```python
from build123d import *

# Parameters (mm, degrees)
SKETCH1_W           = 116
SKETCH1_H           = 79
SKETCH1_W_2         = 112
SKETCH1_H_2         = 75
BOSS_EXTRUDE1_DEPTH = 24
SKETCH2_W           = 116
SKETCH2_H           = 79
BOSS_EXTRUDE2_DEPTH = 2
SKETCH3_W           = 73
SKETCH3_H           = 48
CUT_EXTRUDE1_DEPTH  = 2
SKETCH4_R           = 1.75
CUT_EXTRUDE2_DEPTH  = 2
SKETCH6_R           = 7
CUT_EXTRUDE3_DEPTH  = 10
CUT_EXTRUDE4_DEPTH  = 2
SKETCH8_R           = 5
CUT_EXTRUDE5_DEPTH  = 2


with BuildPart() as part:
    # Sketch1 → Boss-Extrude1 (new body)
    with BuildSketch(Plane(origin=(0, 0, 0), x_dir=(1, 0, 0), z_dir=(0, 1, 0))):
        Rectangle(SKETCH1_W, SKETCH1_H)
        Rectangle(SKETCH1_W_2, SKETCH1_H_2, mode=Mode.SUBTRACT)
    extrude(amount=BOSS_EXTRUDE1_DEPTH)

    # Sketch2 → Boss-Extrude2 (add)
    with BuildSketch(Plane(origin=(0, 24, 0), x_dir=(1, 0, 0), z_dir=(0, 1, 0))):
        Rectangle(SKETCH2_W, SKETCH2_H)
    extrude(amount=BOSS_EXTRUDE2_DEPTH)

    # Sketch3 → Cut-Extrude1 (cut)
    with BuildSketch(Plane(origin=(0, 26, 0), x_dir=(1, 0, 0), z_dir=(0, 1, 0))):
        Rectangle(SKETCH3_W, SKETCH3_H)
    extrude(amount=-CUT_EXTRUDE1_DEPTH, mode=Mode.SUBTRACT)

    # Sketch4 → Cut-Extrude2 (cut)
    with BuildSketch(Plane(origin=(0, 26, 0), x_dir=(1, 0, 0), z_dir=(0, 1, 0))):
        with Locations((50, -27.5)):
            Circle(SKETCH4_R)
    extrude(amount=-CUT_EXTRUDE2_DEPTH, mode=Mode.SUBTRACT)

    # Sketch6 → Cut-Extrude3 (cut)
    with BuildSketch(Plane(origin=(-40.896797153, 42.46975089, 0), x_dir=(-0.720320213, -0.693641687, 0), z_dir=(0.693641687, -0.720320213, 0))):
        with Locations((23.743888519, 0)):
            Circle(SKETCH6_R)
    extrude(amount=CUT_EXTRUDE3_DEPTH, mode=Mode.SUBTRACT)

    # Sketch7 → Cut-Extrude4 (cut)
    with BuildSketch(Plane(origin=(58, 0, 0), x_dir=(0, 0, -1), z_dir=(1, 0, 0))):
        with BuildLine():
            Line((-3.625, 3.5), (-3.625, 0))
            Line((-3.625, 0), (3.625, 0))
            Line((3.625, 0), (3.625, 3.5))
            ThreePointArc((3.625, 3.5), (0, 7.125), (-3.625, 3.5))
        make_face()
    extrude(amount=-CUT_EXTRUDE4_DEPTH, mode=Mode.SUBTRACT)

    # Sketch8 → Cut-Extrude5 (cut)
    with BuildSketch(Plane(origin=(0, 0, -39.5), x_dir=(-1, 0, 0), z_dir=(0, 0, -1))):
        Circle(SKETCH8_R)
    extrude(amount=-CUT_EXTRUDE5_DEPTH, mode=Mode.SUBTRACT)


solid = part.part
```
Source: CAD feature listing. Evaluate the final solid. Frame: model axes, mm. A direction names the side the tool comes from. Give positions to 0.01 mm unless a question says otherwise; leave off trailing zeros. Loops run counter-clockwise (first coordinate to the right, second up) from the corner with the lowest first, then second, coordinate; pieces in that order, holes last. Notation, with made-up numbers: M -2,25.25 L 55,25.25 A33 ccw 55,59.25 Z; hole C -23,30 d10. An arc over 180 degrees is marked long. Put each result on its own line as item: value.
Q1. Section B-B (x = 0). Return the cut outline in (y, z), and give its area (3 significant figures).
Response values:
outline: M 0,37.5 L 24,37.5 L 24,24 L 26,24 L 26,39.5 L 0,39.5 Z; M 5,-39.5 L 26,-39.5 L 26,-24 L 24,-24 L 24,-37.5 L 5,-37.5 Z
area: 148 mm²
Q2. Mould query, pull axis X, two halves, no side actions, for faces 1 (the flat face through (58, 13, 1)), 2 (the flat face through (-58, 13, 1)), 3 (the cylindrical face through (57.014, 7.124, -0.08)), 4 (the cylindrical face through (0, 5, -39)). Classes: released by +X, released by -X, zero draft, split by the parting line, or undercut.
Response values:
face 1: released by +X
face 2: released by -X
face 3: zero draft
face 4: undercut
Q3. Section D-D (z = 0). Return the cut outline in (x, y) (3 decimals).
Response values:
outline: M -58,0 L -56,0 L -56,14.043 L -56.106,13.941 L -58,15.908 Z; M -48.282,26 L -46.356,24 L -36.5,24 L -36.5,26 Z; M 36.5,24 L 56,24 L 56,7.125 L 58,7.125 L 58,26 L 36.5,26 Z
Q4. Pin query (flat end, axial travel): P1, Ø4, axis at x = 27.5, z = 21, coming from the -Y side; P2, Ø8, axis at x = 37.5, z = 7.5, coming from the -Y side; P3, Ø0.6, axis at y = 24.5, z = -5, coming from the -X side. Return the tip coordinate at first contact, or that it passes through.
Response values:
P1: passes through
P2: stops at y = 24
P3: stops at x = -50.29
Q5. Reachability of faces 5 (the flat face through (-26, 0, 38)), 6 (the flat face through (-1, 12, -37.5)) from +Z, -Z, +X, -X, +Y, -Y: full face, straight path, thin tool, end or side. Return the list, or none.
Response values:
face 5: +Z, -Z, +X, -X, -Y
face 6: -Y
Q6. Section A-A (z = 27.5). Return the cut outline in (x, y).
Response values:
outline: M -58,0 L -56,0 L -56,24 L 48.25,24 L 48.25,26 L -58,26 Z; M 51.75,24 L 56,24 L 56,0 L 58,0 L 58,26 L 51.75,26 Z
Q7. Line query: probe 1 along X at (y, z) = (9.25, -30); probe 2 along Z at (x, y) = (50, 25.15); probe 3 along Z at (x, y) = (12, 16). Output: solid intervals per line, ascending. Write a range as [from, to].
Response values:
probe 1: x = [-58, -56], [56, 58]
probe 2: z = [-39.5, 25.75], [29.25, 39.5]
probe 3: z = [-39.5, -37.5], [37.5, 39.5]
Q8. Section C-C (y = 10.25). Return the cut outline in (x, z), and give its area (3 significant figures).
Response values:
outline: M -58,-39.5 L 58,-39.5 L 58,39.5 L -58,39.5 Z; hole M -56,-37.5 L 56,-37.5 L 56,37.5 L -56,37.5 Z
area: 764 mm²
